Verification items for the finished model (mm, model axes). A direction names the side the tool comes from. Give positions to 0.01 mm unless a question says otherwise; leave off trailing zeros. Write each loop counter-clockwise with the first axis right and the second up, starting at its lowest first coordinate (ties: lowest second). Pieces come first, ordered by that corner, then holes. Notation, with made-up numbers: (27, 73.25) -> (75, 73.25) arc R17 cw to (75, 82.25) -> close; hole circle Ø4 at (66, 86.5). An arc over 180 degrees is marked (long way). Use one line per item in the form item = value. Start each with the question number.
(1) Section check A-A, the plane x = 38. Record the cut outline in (y, z) (3 decimals), plus the area to 3 significant figures.
(2) Section check C-C, the plane y = 22. Record the cut outline in (x, z) (3 decimals), plus the area to 3 significant figures.
(3) Scan lines: L1, parallel to Z at x = -15, y = 76.5 (3 decimals); L2, parallel to Z at x = -2, y = -29 (3 decimals); L3, parallel to Z at x = -9, y = 15.5 (3 decimals). Record each from-to range of solid material in increasing order.
(4) Set-up check for faces 4 (the face through (-1.653, 1.245, 66.783)), 5 (the face through (1, 3, -47.625)): record each of +Z, -Z, +X, -X, +Y, -Y from which the full face is reachable in a straight line by a thin tool's end or side.
(5) Section check D-D, the plane x = 23. Record the cut outline in (y, z) (3 decimals).
(6) Release check for a two-part mould opening along Y. For faces 1 (the face through (-30, 3, 0)), 2 (the face through (-1.653, -101.708, 28.931)), 3 (the face through (-19.89, 18.24, -21.91)) record: pulls with the +Y half, pulls with the -Y half, needs draft (parallel to the pull), parting line crosses it, or undercut.
(7) Depth check by flat-ended pin: pin 1 Ø2 at (x, y) = (-16.5, 148.5) entering from +Z (3 decimals); pin 2 Ø10 at (y, z) = (-67, 73) entering from +X; pin 3 Ø1 at (x, z) = (-10.5, 56) entering from +Y. Enter the tip coordinate at first touch or a pass-through.
from build123d import *

# Parameters (mm, degrees)
SKETCH1_R           = 26.9875
BOSS_EXTRUDE1_DEPTH = 44.45
SKETCH2_W           = 88.9
SKETCH2_H           = 381
BOSS_EXTRUDE2_DEPTH = 3.175
SKETCH3_R           = 12.7
SKETCH6_W           = 88.9
SKETCH6_H           = 381
BOSS_EXTRUDE3_DEPTH = 3.175


with BuildPart() as part:
    # Sketch1 → Boss-Extrude1 (new body)
    with BuildSketch(Plane.XY):
        Circle(SKETCH1_R)
    extrude(amount=-BOSS_EXTRUDE1_DEPTH)

    # Sketch2 → Boss-Extrude2 (add)
    with BuildSketch(Plane.XY):
        Rectangle(SKETCH2_W, SKETCH2_H)
    extrude(amount=BOSS_EXTRUDE2_DEPTH)

    # Sweep1: sweep along a path in Sketch5
    with BuildLine(Plane(origin=(0, 0, 0), x_dir=(0, 0, -1), z_dir=(1, 0, 0))) as sweep1_path:
        Line((-3.175, -114.3), (-53.975, -114.3))
        ThreePointArc((-53.975, -114.3), (-71.935512242, -106.860512242), (-79.375, -88.9))
        Line((-79.375, -88.9), (-79.375, 88.9))
        ThreePointArc((-79.375, 88.9), (-71.935512242, 106.860512242), (-53.975, 114.3))
        Line((-53.975, 114.3), (-3.175, 114.3))
    # Sketch3 → Sweep1 (sweep)
    with BuildSketch(Plane.XY.offset(3.175)):
        with Locations((0, -114.3)):
            Circle(SKETCH3_R)
    sweep(path=sweep1_path.line)

    # Sketch6 → Boss-Extrude3 (add)
    with BuildSketch(Plane(origin=(0, 0, -44.45), x_dir=(-1, 0, 0), z_dir=(0, 0, -1))):
        Rectangle(SKETCH6_W, SKETCH6_H)
    extrude(amount=BOSS_EXTRUDE3_DEPTH)


solid = part.part
Completed:
q1.outline = (-190.5, -47.625) -> (190.5, -47.625) -> (190.5, -44.45) -> (-190.5, -44.45) -> close; (-190.5, 0) -> (190.5, 0) -> (190.5, 3.175) -> (-190.5, 3.175) -> close
q1.area = 2,420 mm²
q2.outline = (-44.45, -47.625) -> (44.45, -47.625) -> (44.45, -44.45) -> (15.631, -44.45) -> (15.631, 0) -> (44.45, 0) -> (44.45, 3.175) -> (-44.45, 3.175) -> (-44.45, 0) -> (-15.631, 0) -> (-15.631, -44.45) -> (-44.45, -44.45) -> close; circle Ø25.4 at (0, 79.375)
q2.area = 2,460 mm²
q3.L1 = -47.625 to -44.45, 0 to 3.175
q3.L2 = -47.625 to -44.45, 0 to 3.175, 66.833 to 91.917
q3.L3 = -47.625 to 3.175, 70.415 to 88.335
q4.face_4 = none
q4.face_5 = -Z, +X, -X, +Y, -Y
q5.outline = (-190.5, -47.625) -> (190.5, -47.625) -> (190.5, -44.45) -> (14.118, -44.45) -> (14.118, 0) -> (190.5, 0) -> (190.5, 3.175) -> (-190.5, 3.175) -> (-190.5, 0) -> (-14.118, 0) -> (-14.118, -44.45) -> (-190.5, -44.45) -> close
q6.face_1 = needs draft
q6.face_2 = undercut
q6.face_3 = parting line crosses it
q7.pin_1 = 3.175
q7.pin_2 = 12.63
q7.pin_3 = 122.07
